For this review, use the dimensioned drawing (mm, ordinates from the lowest corner) and the shaded views. Coordinates: 2 decimals unless noted, no trailing zeros. Order: outer loops, then holes, each group sorted by start corner. A loop starts at its lowest first (then second) coordinate and runs counter-clockwise, first axis right, second up. Notation, with made-up numbers: M 47,87 L 51,87 A21 ccw 51,100 Z; hole C -33,27.5 d4. An arc over 180 degrees is marked long. Answer as CSV lines item,"result". Start each with the question number.
Q1. Consider section D-D on z = 177.8. Write out the cut boundary in (x, y) (3 decimals), and give its area (3 significant figures).
Q2. Consider section C-C on x = 127. Write out the cut boundary in (y, z) (3 decimals).
Q3. Consider section B-B on z = 82.55. Write out the cut boundary in (x, y) (3 decimals), and give its area (3 significant figures).
Q4. Wall thickness on L1, parallel to X at y = 7.5, z = 177.8 (3 decimals); L2, parallel to X at y = 4.5, z = 82.55 (3 decimals); L3, parallel to X at y = 1.25, z = 85: over which ranges is each line inside the solid? List them lowest first. Write a range as [from, to].
Q5. Consider section A-A on x = 330.2. Write out the cut boundary in (y, z) (3 decimals).
Q6. For P1, Ø11.5, axis at x = 330.2, z = 82.55, coming from the -Y side; P2, Ø6, axis at x = 390, z = 243.5, coming from the -Y side, all flat-tipped, find the tip position at first contact; note any pin that passes through.
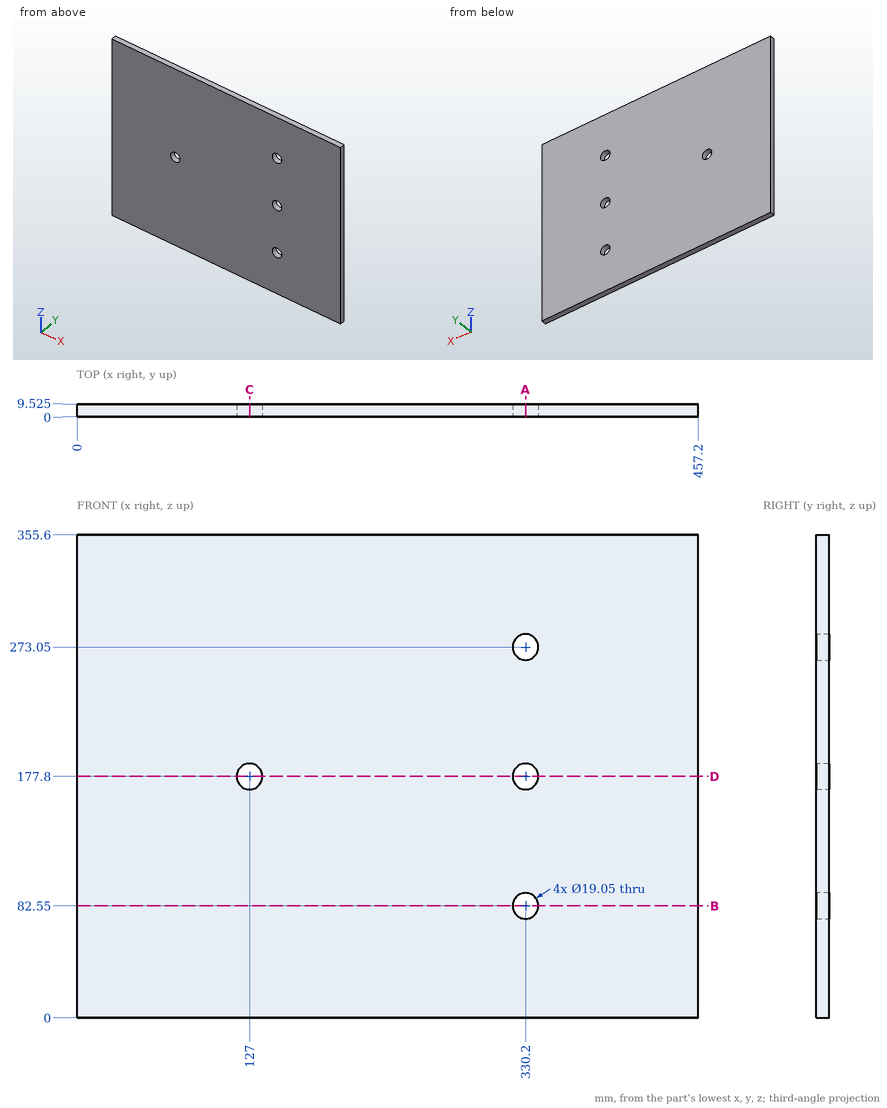
Evaluation:
1,outline,"M 0,0 L 117.475,0 L 117.475,9.525 L 0,9.525 Z; M 136.525,0 L 320.675,0 L 320.675,9.525 L 136.525,9.525 Z; M 339.725,0 L 457.2,0 L 457.2,9.525 L 339.725,9.525 Z"
1,area,"3,990 mm²"
2,outline,"M 0,0 L 9.525,0 L 9.525,168.275 L 0,168.275 Z; M 0,187.325 L 9.525,187.325 L 9.525,355.6 L 0,355.6 Z"
3,outline,"M 0,0 L 320.675,0 L 320.675,9.525 L 0,9.525 Z; M 339.725,0 L 457.2,0 L 457.2,9.525 L 339.725,9.525 Z"
3,area,"4,170 mm²"
4,L1,"x = [0, 117.475], [136.525, 320.675], [339.725, 457.2]"
4,L2,"x = [0, 320.675], [339.725, 457.2]"
4,L3,"x = [0, 321], [339.4, 457.2]"
5,outline,"M 0,0 L 9.525,0 L 9.525,73.025 L 0,73.025 Z; M 0,92.075 L 9.525,92.075 L 9.525,168.275 L 0,168.275 Z; M 0,187.325 L 9.525,187.325 L 9.525,263.525 L 0,263.525 Z; M 0,282.575 L 9.525,282.575 L 9.525,355.6 L 0,355.6 Z"
6,P1,"passes through"
6,P2,"stops at y = 0"
